Can you work these out from the model? Positions are in its coordinate system, mm. A direction names the side the tool comes from. Round coordinates to 2 decimals unless told otherwise and drop trailing zeros. Write each loop counter-clockwise with the first axis right and the second up, starting at its lowest first coordinate (ties: lowest second). Pieces come first, ordered by that corner, then holes. Notation, with made-up numbers: M -33,36.5 L -21,36.5 A15 cw -21,54.5 Z; hole C 19,1 d1. An arc over 180 degrees is marked long. Answer in a Markdown table with one row per item. Add a question column.
(1) I'm going to push flat-ended pins straight in: pin 1 (1.5 mm diameter, centred on x = 269, y = 19, fed in from -Z); pin 2 (4 mm diameter, centred on x = 223, y = -40, fed in from -Z); pin 3 (1.5 mm diameter, centred on x = 291, y = -28, fed in from +Z); pin 4 (24 mm diameter, centred on y = 0, z = -60, fed in from -X). Where does each tip first touch, or does it pass through?
(2) For faces 1 (the face through (-11.34, -13.41, -27.67)), 2 (the face through (311, -21, -32)), 3 (the face through (152.1, 19.594, 105.596)), which set-ups out of +Z, -Z, +X, -X, +Y, -Y let a thin tool reach every point of the face, with its end or its side?
(3) Suppose I cut it at B-B, the plane x = 137. Write out the boundary of the cut face in (y, z).
(4) If we mould it in two halves opening along Z, with no side actions, what happens to faces 4 (the face through (147.9, 0.66, 45.015)), 5 (the face through (147.9, 43.26, 85.07)), 6 (the face through (147.9, -42.882, -85.713))? For each: released by +Z, released by -Z, zero draft, split by the parting line, or undercut.
(5) Suppose I cut it at D-D, the plane z = -2. Write out the boundary of the cut face in (x, y).
(6) Suppose I cut it at A-A, the plane y = 0. Write out the boundary of the cut face in (x, z), then the cut area to 3 significant figures.
(7) Suppose I cut it at C-C, the plane x = -6. Write out the boundary of the cut face in (y, z), then the cut area to 3 significant figures.
(8) If I drill on probe 1 along Y at (x, z) = (78, 60); probe 2 along Z at (x, y) = (47.5, 11.5); probe 3 along Z at (x, y) = (51, 6), over which ranges is the centre line in solid material (lowest first)?
from build123d import *

# Parameters (mm, degrees)
SKETCH_2_W          = 120
SKETCH_2_H          = 100
EXTRUDE_1_DEPTH     = 300
SKETCH_3_R          = 15
CUT_EXTRUDE_1_DEPTH = 300
SKETCH_4_R          = 35
SKETCH_4_R_2        = 15
EXTRUDE_2_DEPTH     = 28
SKETCH_6_R          = 35
SKETCH_6_R_2        = 15
EXTRUDE_3_DEPTH     = 28
FILLET_2_R          = 5
FILLET_3_R          = 20


with BuildPart() as part:
    # 草图2 → 凸台-拉伸1 (new body)
    with BuildSketch(Plane(origin=(0, 0, 0), x_dir=(0, 0, -1), z_dir=(1, 0, 0))):
        with BuildLine():
            Line((106.249324319, 19), (106.249324319, -19))
            ThreePointArc((106.249324319, -19), (10, 0), (106.249324319, 19))
        make_face()
        Rectangle(SKETCH_2_W, SKETCH_2_H)
        with BuildLine():
            Line((-106.249324319, 19), (-106.249324319, -19))
            ThreePointArc((-106.249324319, -19), (-10, 0), (-106.249324319, 19))
        make_face()
    extrude(amount=EXTRUDE_1_DEPTH)

    # 草图3 → 切除-拉伸1 (cut)
    with BuildSketch(Plane.ZY):
        with Locations((60, 0)):
            Circle(SKETCH_3_R)
        with Locations((-60, 0)):
            Circle(SKETCH_3_R)
    extrude(amount=-CUT_EXTRUDE_1_DEPTH, mode=Mode.SUBTRACT)

    # 草图4 → 凸台-拉伸2 (add)
    with BuildSketch(Plane.ZY):
        with Locations((-60, 0)):
            Circle(SKETCH_4_R)
        with Locations((-60, 0)):
            Circle(SKETCH_4_R_2, mode=Mode.SUBTRACT)
    extrude(amount=EXTRUDE_2_DEPTH)

    # 草图6 → 凸台-拉伸3 (add)
    with BuildSketch(Plane(origin=(300, 0, 0), x_dir=(0, 0, -1), z_dir=(1, 0, 0))):
        with Locations((60, 0)):
            Circle(SKETCH_6_R)
        with Locations((60, 0)):
            Circle(SKETCH_6_R_2, mode=Mode.SUBTRACT)
    extrude(amount=EXTRUDE_3_DEPTH)

    # 圆角2
    fillet_2_edges = [part.edges().sort_by_distance(p)[0] for p in [
        (-28, 0, -95),
        (328, 0, -25),
    ]]
    fillet(fillet_2_edges, radius=FILLET_2_R)

    # 圆角3
    fillet_3_edges = [part.edges().sort_by_distance(p)[0] for p in [
        (150, -19, 106.249324319),
        (150, 19, 106.249324319),
        (150, 19, -106.249324319),
        (150, -19, -106.249324319),
    ]]
    fillet(fillet_3_edges, radius=FILLET_3_R)


solid = part.part
Calculated:
| question | item | result |
|---|---|---|
| 1 | pin 1 | z = -105.9 |
| 1 | pin 2 | z = -92.5 |
| 1 | pin 3 | z = 101.92 |
| 1 | pin 4 | through |
| 2 | face 1 | -X |
| 2 | face 2 | +X |
| 2 | face 3 | +Z, +X, -X, +Y |
| 3 | outline | M -50,-60 A50 ccw -24.21,-103.75 A20 ccw -14.52,-106.25 L 14.52,-106.25 A20 ccw 24.21,-103.75 A50 ccw 50,-60 L 50,60 A50 ccw 24.21,103.75 A20 ccw 14.52,106.25 L -14.52,106.25 A20 ccw -24.21,103.75 A50 ccw -50,60 Z; hole C 0,-60 d30; hole C 0,60 d30 |
| 4 | face 4 | undercut |
| 4 | face 5 | released by +Z |
| 4 | face 6 | released by -Z |
| 5 | outline | M 0,-50 L 300,-50 L 300,50 L 0,50 Z |
| 6 | outline | M -28,-90 A5 ccw -23,-95 L 0,-95 L 0,-106.25 L 300,-106.25 L 300,-95 L 323,-95 A5 ccw 328,-90 L 328,-75 L -28,-75 Z; M -28,-45 L 328,-45 L 328,-30 A5 ccw 323,-25 L 300,-25 L 300,45 L 0,45 L 0,-25 L -23,-25 A5 ccw -28,-30 Z; M 0,75 L 300,75 L 300,106.25 L 0,106.25 Z |
| 6 | area | 48,000 mm² |
| 7 | outline | C 0,-60 d70; hole C 0,-60 d30 |
| 7 | area | 3,140 mm² |
| 8 | probe 1 | -50 to -15, 15 to 50 |
| 8 | probe 2 | -106.25 to -69.63, -50.37 to 50.37, 69.63 to 106.25 |
| 8 | probe 3 | -106.25 to -73.75, -46.25 to 46.25, 73.75 to 106.25 |
